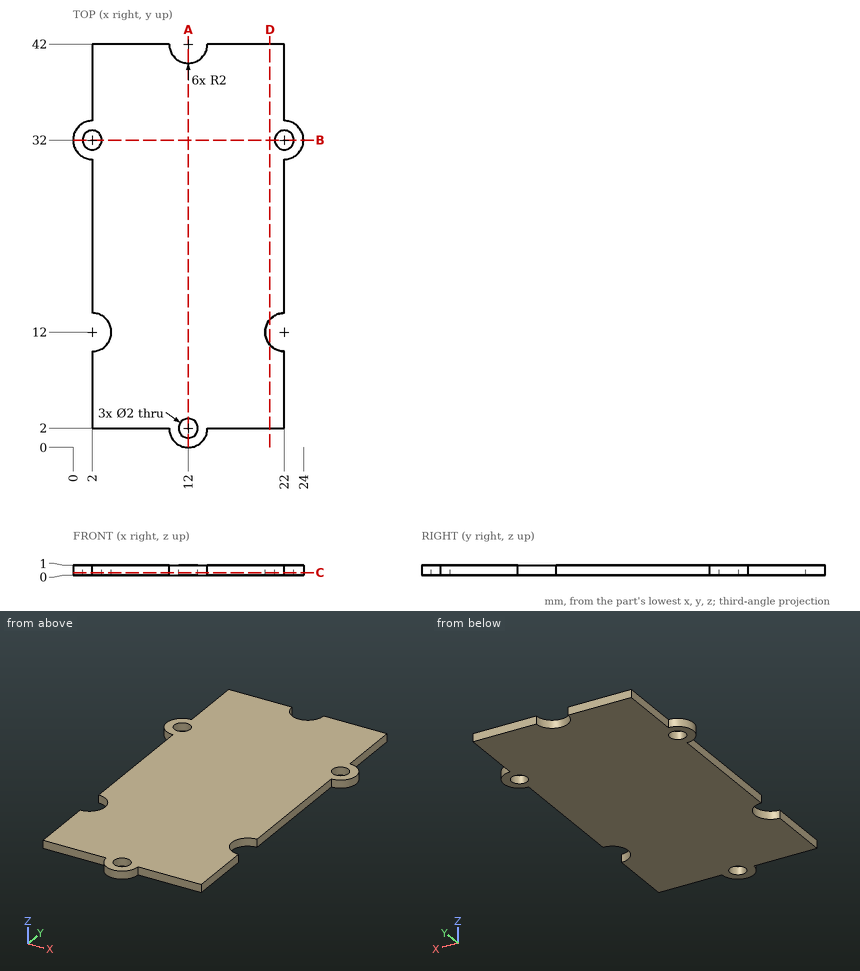
Job drawing, mm, ordinate dimensions from the low corner. One solid piece. Coordinates: 2 decimals unless noted, no trailing zeros. Write each loop counter-clockwise with the first axis right and the second up, starting at its lowest first coordinate (ties: lowest second). Pieces come first, ordered by that corner, then holes. Notation, with made-up numbers: (9.5, 64.5) -> (35.5, 64.5) arc R24 ccw to (35.5, 96.5) -> close; hole circle Ø3 at (25, 83). An arc over 180 degrees is marked (long way). Use CSV: the item, a comma, the result in double quotes. Start each with the question number.
Item 1: Wall check: probe 1 along X at (y, z) = (32, 0.75); probe 2 along Y at (x, z) = (12, 0.1); probe 3 along X at (y, z) = (32.5, 0.6). Give the ranges that are in metal, low to high.
Item 2: Band-saw the part on A-A, the plane x = 12. Write the cut outline in (y, z), plus the area to 3 significant figures.
Item 3: Band-saw the part on C-C, the plane z = 0.25. Write the cut outline in (x, y), plus the area to 3 significant figures.
Item 4: Band-saw the part on B-B, the plane y = 32. Write the cut outline in (x, z).
Item 5: Band-saw the part on D-D, the plane x = 20.5. Write the cut outline in (y, z).
Item 6: Drop flat-ended pins along their axis: P1, Ø0.5, axis at y = 37.5, z = 0.5, coming from the -X side; P2, Ø2.5, axis at x = 22, y = 32, coming from the +Z side; P3, Ø0.5, axis at x = 6, z = 0.5, coming from the -Y side. Give the stop position or say it passes through.
Response values:
1,probe 1,"x = 0 to 1, 3 to 21, 23 to 24"
1,probe 2,"y = 0 to 1, 3 to 40"
1,probe 3,"x = 0.06 to 1.13, 2.87 to 21.13, 22.87 to 23.94"
2,outline,"(0, 0) -> (1, 0) -> (1, 1) -> (0, 1) -> close; (3, 0) -> (40, 0) -> (40, 1) -> (3, 1) -> close"
2,area,"38.0 mm2"
3,outline,"(2, 2) -> (10, 2) arc R2 ccw to (14, 2) -> (22, 2) -> (22, 10) arc R2 cw to (22, 14) -> (22, 30) arc R2 ccw to (22, 34) -> (22, 42) -> (14, 42) arc R2 cw to (10, 42) -> (2, 42) -> (2, 34) arc R2 ccw to (2, 30) -> (2, 14) arc R2 cw to (2, 10) -> close; hole circle Ø2 at (2, 32); hole circle Ø2 at (12, 2); hole circle Ø2 at (22, 32)"
3,area,"791 mm2"
4,outline,"(0, 0) -> (1, 0) -> (1, 1) -> (0, 1) -> close; (3, 0) -> (21, 0) -> (21, 1) -> (3, 1) -> close; (23, 0) -> (24, 0) -> (24, 1) -> (23, 1) -> close"
5,outline,"(2, 0) -> (10.68, 0) -> (10.68, 1) -> (2, 1) -> close; (13.32, 0) -> (42, 0) -> (42, 1) -> (13.32, 1) -> close"
6,P1,"stops at x = 2"
6,P2,"stops at z = 1"
6,P3,"stops at y = 2"
